```python
from build123d import *

# Parameters (mm, degrees)
F0_R     = 11.225
F1_DEPTH = 7
F2_R     = 25
F3_R     = 1.5


with BuildPart() as f1:
    # F0 (on Top) → F1 (new body)
    with BuildSketch(Plane.XY):
        with BuildLine():
            Line((-14.0909507949, -16.6224631917), (-8.8518149883, -13.5976467234))
            ThreePointArc((-8.8518149883, -13.5976467234), (0, -16.225), (8.8518149883, -13.5976467234))
            Line((8.8518149883, -13.5976467234), (14.0909507949, -16.6224631917))
            ThreePointArc((14.0909507949, -16.6224631917), (36.3730669589, -21), (21.4409507949, -3.8918897561))
            Line((21.4409507949, -3.8918897561), (16.2018149883, -0.8670732877))
            ThreePointArc((16.2018149883, -0.8670732877), (14.0512621764, 8.1125), (7.35, 14.4647200111))
            Line((7.35, 14.4647200111), (7.35, 20.5143529477))
            ThreePointArc((7.35, 20.5143529477), (0, 42), (-7.35, 20.5143529477))
            Line((-7.35, 20.5143529477), (-7.35, 14.4647200111))
            ThreePointArc((-7.35, 14.4647200111), (-14.0512621764, 8.1125), (-16.2018149883, -0.8670732877))
            Line((-16.2018149883, -0.8670732877), (-21.4409507949, -3.8918897561))
            ThreePointArc((-21.4409507949, -3.8918897561), (-36.3730669589, -21), (-14.0909507949, -16.6224631917))
        make_face()
        Polygon((-25.9807621135, -23.4870489571), (-33.3307621135, -19.2435244785), (-33.3307621135, -10.7564755215), (-25.9807621135, -6.5129510429), (-18.6307621135, -10.7564755215), (-18.6307621135, -19.2435244785), align=None, mode=Mode.SUBTRACT)
        Circle(F0_R, mode=Mode.SUBTRACT)
        Polygon((33.3307621135, -10.7564755215), (33.3307621135, -19.2435244785), (25.9807621135, -23.4870489571), (18.6307621135, -19.2435244785), (18.6307621135, -10.7564755215), (25.9807621135, -6.5129510429), align=None, mode=Mode.SUBTRACT)
        Polygon((0, 38.4870489571), (7.35, 34.2435244785), (7.35, 25.7564755215), (0, 21.5129510429), (-7.35, 25.7564755215), (-7.35, 34.2435244785), align=None, mode=Mode.SUBTRACT)
        with BuildLine():
            Line((-7.35, 20.5143529477), (-21.4409507949, -3.8918897561))
            Line((-21.4409507949, -3.8918897561), (-16.2018149883, -0.8670732877))
            ThreePointArc((-16.2018149883, -0.8670732877), (-14.0512621764, 8.1125), (-7.35, 14.4647200111))
            Line((-7.35, 14.4647200111), (-7.35, 20.5143529477))
        make_face()
        with BuildLine():
            Line((16.2018149883, -0.8670732877), (21.4409507949, -3.8918897561))
            Line((21.4409507949, -3.8918897561), (7.35, 20.5143529477))
            Line((7.35, 20.5143529477), (7.35, 14.4647200111))
            ThreePointArc((7.35, 14.4647200111), (14.0512621764, 8.1125), (16.2018149883, -0.8670732877))
        make_face()
        with BuildLine():
            ThreePointArc((8.8518149883, -13.5976467234), (0, -16.225), (-8.8518149883, -13.5976467234))
            Line((-8.8518149883, -13.5976467234), (-14.0909507949, -16.6224631917))
            Line((-14.0909507949, -16.6224631917), (14.0909507949, -16.6224631917))
            Line((14.0909507949, -16.6224631917), (8.8518149883, -13.5976467234))
        make_face()
    extrude(amount=F1_DEPTH)

    # F2
    f2_edges = [f1.edges().sort_by_distance(p)[0] for p in [
        (-21.440951, -3.89189, 3.5),
        (7.35, 20.514353, 3.5),
        (14.090951, -16.622463, 3.5),
        (21.440951, -3.89189, 3.5),
        (-7.35, 20.514353, 3.5),
        (-14.090951, -16.622463, 3.5),
    ]]
    fillet(f2_edges, radius=F2_R)

    # F3
    f3_edges = [f1.edges().sort_by_distance(p)[0] for p in [
        (-11.147106, 17.57587, 7),
        (-20.794703, 0.865742, 7),
        (-36.373067, -21, 7),
        (-9.647597, -18.441612, 7),
        (36.373067, -21, 7),
        (20.794703, 0.865742, 7),
        (11.147106, 17.57587, 7),
        (0, 42, 7),
        (0, 42, 0),
        (-11.147106, 17.57587, 0),
        (-20.794703, 0.865742, 0),
        (-36.373067, -21, 0),
        (-9.647597, -18.441612, 0),
        (9.647597, -18.441612, 0),
        (36.373067, -21, 0),
        (20.794703, 0.865742, 0),
        (0, -16.622463, 0),
        (14.395475, 8.311232, 0),
        (11.147106, 17.57587, 0),
        (-14.395475, 8.311232, 0),
        (9.647597, -18.441612, 7),
        (0, -16.622463, 7),
        (14.395475, 8.311232, 7),
        (-14.395475, 8.311232, 7),
    ]]
    fillet(f3_edges, radius=F3_R)


solid = f1.part
```
For this review, take the finished solid that the model builds, in its own axes (mm). A direction names the side the tool comes from. Give positions to 0.01 mm unless a question says otherwise; leave off trailing zeros.
Item 1: Take a section at A-A (z = 4.5). Give the number of separate pieces and of enclosed holes in the cut face, and give its area (3 significant figures).
Item 2: Insertion check: P1, Ø3, axis at y = 1, z = 4.5, coming from the -X side; P2, Ø4, axis at y = 29.5, z = 5, coming from the +X side; P3, Ø2, axis at y = 25.5, z = 6.5, coming from the -X side. Each pin has a flat end and moves straight along its axis. Give the tip position at first contact, or say it passes through.
Item 3: Machinability: for faces 1 (the face through (20.901, 0.783, 3.528)), 2 (the face through (-29.707, -8.664, 3.451)), 3 (the face through (-9.77, -18.49, 3.53)), which of the approach directions +Z, -Z, +X, -X, +Y, -Y give a long, thin tool a straight path to every point of the face, cutting with its end or side? Answer none if there is none.
Item 4: The part is to be moulded in two halves that separate along Y. For faces 4 (the face through (-11, 3, 7)), 5 (the face through (36.22, -21.26, 3.47)), 6 (the face through (-22.357, -8.605, 3.451)), say which applies: +Y half, -Y half, draft (parallel to the pull), parting line (faces both ways), or undercut.
Item 5: Wall thickness on probe 1 along Y at (x, z) = (0, 5) (3 decimals); probe 2 along X at (y, z) = (29.5, 4.75); probe 3 along X at (y, z) = (-11.5, 4.75): over which ranges is each line inside the solid? List them lowest first.
Established:
1. separate pieces: 1
1. enclosed holes: 4
1. area: 1,610 mm2
2. P1: stops at x = -22.72
2. P2: stops at x = 12
2. P3: stops at x = -11.41
3. face 1: +Z, -Z, +X, +Y
3. face 2: +Z, -Z
3. face 3: +Z, -Z, -Y
4. face 4: draft
4. face 5: parting line
4. face 6: undercut
5. probe 1: y = -16.622 to -11.225, 11.225 to 21.513, 38.487 to 42
5. probe 2: x = -11.99 to -7.35, 7.35 to 11.99
5. probe 3: x = -37.46 to -33.33, -18.63 to 18.63, 33.33 to 37.46
